from build123d import *

# Parameters (mm, degrees)
SKETCH1_W           = 30
SKETCH1_H           = 15
BOSS_EXTRUDE1_DEPTH = 3
SKETCH2_W           = 20
SKETCH2_H           = 10
CUT_EXTRUDE1_DEPTH  = 18.036725037
BOSS_EXTRUDE2_DEPTH = 3


with BuildPart() as part:
    # Sketch1 → Boss-Extrude1 (new body)
    with BuildSketch(Plane.XY):
        Rectangle(SKETCH1_W, SKETCH1_H)
    extrude(amount=BOSS_EXTRUDE1_DEPTH)

    # Sketch2 → Cut-Extrude1 (cut, through all)
    with BuildSketch(Plane.XY.offset(3)):
        Rectangle(SKETCH2_W, SKETCH2_H)
    extrude(amount=-CUT_EXTRUDE1_DEPTH, mode=Mode.SUBTRACT)

    # Sketch3 → Boss-Extrude2 (add)
    # profile 1 of 3: a face of its own
    with BuildSketch(Plane.XY.offset(3)):
        Polygon((-8.717948718, 5), (-3.846153846, 5), (-3.846153846, 3.974358974), (-7.820512821, 3.974358974), (-7.820512821, 0.897435897), (-3.846153846, 0.897435897), (-3.846153846, -0.128205128), (-7.820512821, -0.128205128), (-7.820512821, -5), (-8.717948718, -5), align=None)
    # profile 2 of 3: a face of its own
    with BuildSketch(Plane.XY.offset(3)):
        with BuildLine():
            Line((-2.897435897, 5), (-0.896233974, 5))
            add(Edge.make_bspline(
                [(-0.896233974, 5), (-0.762687893, 4.999555469), (-0.506264623, 4.998701919), (-0.138912422, 4.993942596), (0.194879284, 4.98030158), (0.494935967, 4.96856277), (0.761252124, 4.947157224), (0.994644384, 4.926698232), (1.194037805, 4.899916344), (1.314740237, 4.875043707), (1.369391026, 4.863782051)],
                knots=[0, 0, 0, 0, 1.410062039, 2.707475311, 3.878576406, 4.937260626, 5.877586885, 6.699081471, 7.410979367, 8, 8, 8, 8], degree=3))
            add(Edge.make_bspline(
                [(1.369391026, 4.863782051), (1.442552809, 4.845705579), (1.587315636, 4.809938254), (1.795744396, 4.734339395), (1.99435675, 4.646854753), (2.182327677, 4.544101266), (2.358715652, 4.425316181), (2.525339397, 4.292550117), (2.682955006, 4.146529529), (2.825188236, 3.983572839), (2.959299812, 3.812611383), (3.072410173, 3.627743506), (3.169914401, 3.434424856), (3.24754445, 3.230689377), (3.310052945, 3.018512886), (3.354127915, 2.795973467), (3.38055988, 2.564084967), (3.383250895, 2.405919513), (3.384615385, 2.325721154)],
                knots=[0, 0, 0, 0, 1.027469482, 2.033020251, 3.019912614, 3.986113645, 4.951240523, 5.91722682, 6.890402269, 7.87763091, 8.8651537, 9.85103654, 10.82876324, 11.815024772, 12.821070561, 13.842952187, 14.906261191, 16, 16, 16, 16], degree=3))
            add(Edge.make_bspline(
                [(3.384615385, 2.325721154), (3.380418247, 2.192477998), (3.372228545, 1.93248609), (3.295871106, 1.555169286), (3.170795335, 1.203199815), (2.998443081, 0.87702085), (2.778958865, 0.582990434), (2.515173747, 0.324731991), (2.206940571, 0.108617955), (1.919999669, -0.041247202), (1.666530527, -0.137226941), (1.457863919, -0.204759394), (1.230243983, -0.256936438), (0.985851598, -0.303679672), (0.723669726, -0.338970227), (0.444326756, -0.36481764), (0.147623466, -0.380972065), (-0.056202447, -0.383377793), (-0.161057692, -0.384615385)],
                knots=[0, 0, 0, 0, 1.260483769, 2.459530307, 3.627416485, 4.787058657, 5.939039949, 7.08810263, 8.267026773, 9.491475466, 10.141966685, 10.831826277, 11.566392101, 12.351337768, 13.187381173, 14.07005841, 15.007169909, 16, 16, 16, 16], degree=3))
            Line((-0.161057692, -0.384615385), (3.512820513, -5))
            Line((3.512820513, -5), (2.403044872, -5))
            Line((2.403044872, -5), (-1.270833333, -0.384615385))
            Line((-1.270833333, -0.384615385), (-2, -0.384615385))
            Line((-2, -0.384615385), (-2, -5))
            Line((-2, -5), (-2.897435897, -5))
            Line((-2.897435897, -5), (-2.897435897, 5))
        make_face()
        with BuildLine():
            Line((-2, 3.974358974), (-2, 0.641025641))
            Line((-2, 0.641025641), (-0.169070513, 0.627003205))
            add(Edge.make_bspline(
                [(-0.169070513, 0.627003205), (-0.083584687, 0.626965386), (0.08211119, 0.626892082), (0.321827375, 0.638302871), (0.545027694, 0.651283781), (0.750858415, 0.671139054), (0.939411487, 0.69672783), (1.110592668, 0.728736356), (1.264681388, 0.766027964), (1.444391497, 0.823746895), (1.645067301, 0.915192661), (1.863157187, 1.048236943), (2.048878152, 1.215577284), (2.20578633, 1.406930015), (2.33187042, 1.617319298), (2.420762003, 1.84422321), (2.477168981, 2.08191349), (2.483821968, 2.245279512), (2.487179487, 2.327724359)],
                knots=[0, 0, 0, 0, 1.146690395, 2.22261258, 3.21895312, 4.145990853, 4.996080663, 5.770904154, 6.481378293, 7.121626537, 8.300444488, 9.431385265, 10.535395872, 11.636531494, 12.74115979, 13.810798291, 14.895190096, 16, 16, 16, 16], degree=3))
            add(Edge.make_bspline(
                [(2.487179487, 2.327724359), (2.483744855, 2.408143141), (2.476938669, 2.567503823), (2.421370759, 2.800806424), (2.327401098, 3.02099771), (2.200766132, 3.227181953), (2.046482832, 3.414341198), (1.865574796, 3.574475921), (1.662988524, 3.706617249), (1.473642243, 3.791058336), (1.304401636, 3.842829345), (1.15745975, 3.879261242), (0.991426957, 3.908531153), (0.805497075, 3.931982755), (0.600463844, 3.952139739), (0.375290555, 3.96571625), (0.131471183, 3.973755861), (-0.037520049, 3.974153258), (-0.125, 3.974358974)],
                knots=[0, 0, 0, 0, 1.101028733, 2.181837193, 3.264309656, 4.369019818, 5.486613113, 6.575447106, 7.666700264, 8.788928104, 9.402425223, 10.0903467, 10.862060571, 11.710948788, 12.657782767, 13.684531032, 14.801375019, 16, 16, 16, 16], degree=3))
            Line((-0.125, 3.974358974), (-2, 3.974358974))
        make_face(mode=Mode.SUBTRACT)
    # profile 3 of 3: a face of its own
    with BuildSketch(Plane.XY.offset(3)):
        Polygon((4.717948718, 5), (5.615384615, 5), (5.615384615, -3.974358974), (9.461538462, -3.974358974), (9.461538462, -5), (4.717948718, -5), align=None)
    extrude(amount=-BOSS_EXTRUDE2_DEPTH)


solid = part.part
Verification items for the finished model (mm, model axes). A direction names the side the tool comes from. Give positions to 0.01 mm unless a question says otherwise; leave off trailing zeros. Loops run counter-clockwise (first coordinate to the right, second up) from the corner with the lowest first, then second, coordinate; pieces in that order, holes last. Notation, with made-up numbers: (-31.75, 25) - (20.25, 25) arc R26 cw to (20.25, 47) - close; hole circle Ø6 at (-22, 73.5). An arc over 180 degrees is marked (long way). Write item = value, one per line. Start each with the question number.
Q1. Tool access check on faces 1 (the face through (0, 0, 0)), 2 (the face through (-3.846, 4.5, 1.5)). Record the directions out of +Z, -Z, +X, -X, +Y, -Y that give a thin tool (end or side, any length) a straight path to the whole face; none if there is none.
Q2. Cross-section at B-B, the plane z = 1. State how many separate pieces and enclosed holes the cut face has, and give its area (3 significant figures).
Q3. Cross-section at A-A, the plane y = -2.25. Enter the section's corners in (x, z).
Q4. Thickness scan on line 1 (Y direction, x = -4.5, z = 2.5); line 2 (Y direction, x = 7.5, z = 1.6); line 3 (X direction, y = 2.25, z = 2.65). Record the ranges inside material, lowest first.
Q5. Mould release check, pull along X, two halves, no side actions. Record for faces 3 (the face through (0, 0, 3)), 4 (the face through (4, -5, 2)), 5 (the face through (15, 0, 1)): released by +X, released by -X, zero draft, split by the parting line, or undercut.
Answer key:
q1.face_1 = -Z, +X, -X, +Y, -Y
q1.face_2 = +Z, -Z
q2.separate_pieces = 1
q2.enclosed_holes = 6
q2.area = 306 mm^2
q3.outline = (-15, 0) - (-10, 0) - (-10, 3) - (-15, 3) - close; (-8.72, 0) - (-7.82, 0) - (-7.82, 3) - (-8.72, 3) - close; (-2.9, 0) - (-2, 0) - (-2, 3) - (-2.9, 3) - close; (0.21, 0) - (1.32, 0) - (1.32, 3) - (0.21, 3) - close; (4.72, 0) - (5.62, 0) - (5.62, 3) - (4.72, 3) - close; (10, 0) - (15, 0) - (15, 3) - (10, 3) - close
q4.line_1 = -7.5 to -5, -0.13 to 0.9, 3.97 to 7.5
q4.line_2 = -7.5 to -3.97, 5 to 7.5
q4.line_3 = -15 to -10, -8.72 to -7.82, -2.9 to -2, 2.48 to 3.38, 4.72 to 5.62, 10 to 15
q5.face_3 = zero draft
q5.face_4 = undercut
q5.face_5 = released by +X
